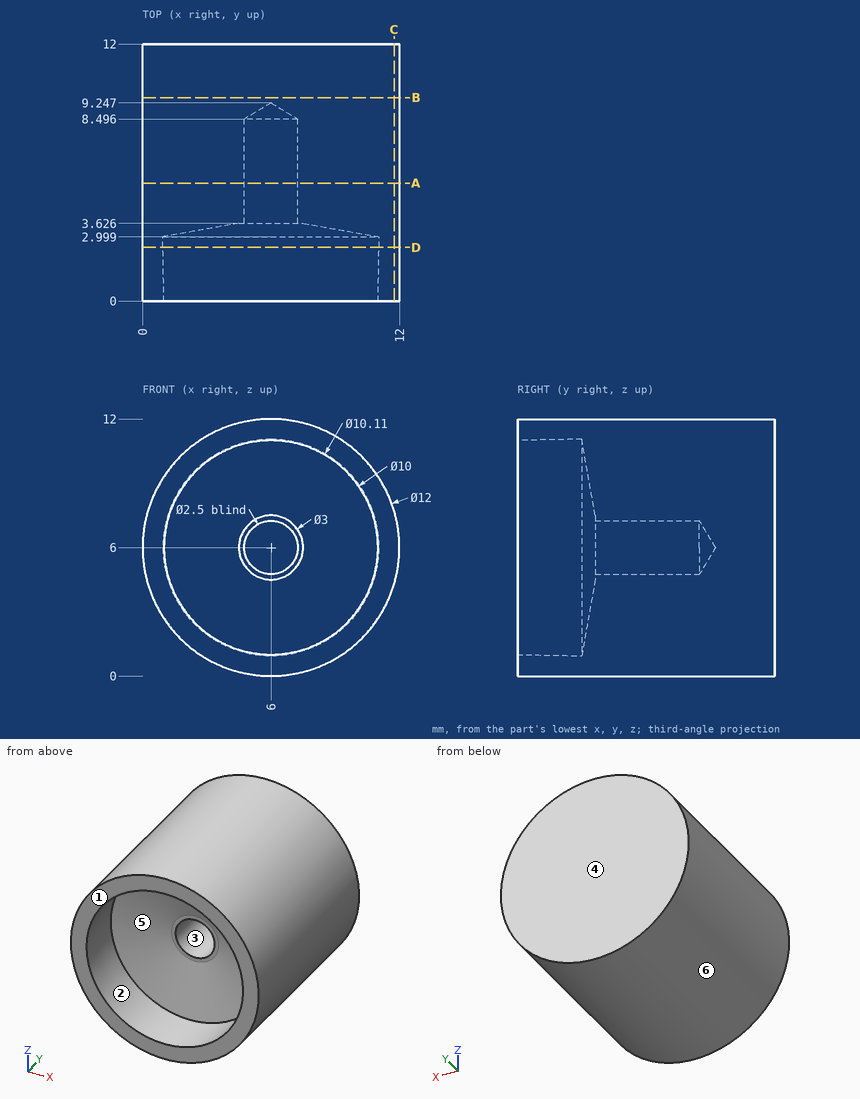
Input: dimensioned drawing with shaded views. Units: mm. Origin: part minimum x, y, z. A direction names the side the tool comes from. Coordinates: 2 decimals unless noted, no trailing zeros. Loops run counter-clockwise (first coordinate to the right, second up) from the corner with the lowest first, then second, coordinate; pieces in that order, holes last. Notation, with made-up numbers: M 74,80.5 L 85,80.5 A27 cw 85,103.5 Z; hole C 79,73 d8. An arc over 180 degrees is marked long. Use a Markdown table: item, result. Add a question column.
1) Section C-C, the plane x = 11.75. Return the cut outline in (y, z).
2) Section A-A, the plane y = 5.5. Return the cut outline in (x, z).
3) Set-up query: the marked faces 1 and 2. Return all of +Z, -Z, +X, -X, +Y, -Y with unobstructed straight access to the full face (end or side cutting, diameter ignored); none if empty.
4) Line query: L1, parallel to X at y = 5.1, z = 6; L2, parallel to X at y = 2.5, z = 10 (1 decimal). Output: solid intervals per line, ascending. Write a range as from..to.
5) Draft query along Z for the marked faces 3, 4, 5 and 6. Return one class per face: +Z half, -Z half, draft (parallel to the pull), parting line (faces both ways), or undercut.
6) Section D-D, the plane y = 2.5. Return the cut outline in (x, z) (1 decimal).
7) Section B-B, the plane y = 9.5. Return the cut outline in (x, z).
8) Pin query (flat end, axial travel): P1, Ø2.5, axis at x = 6.5, z = 6, coming from the -Y side; P2, Ø1.5, axis at x = 10, y = 6.5, coming from the +Z side (1 decimal); P3, Ø1, axis at x = 8.5, y = 1.5, coming from the -Z side. Return the tip coordinate at first contact, or that it passes through.
Answer below:
| question | item | result |
|---|---|---|
| 1 | outline | M 0,4.29 L 12,4.29 L 12,7.71 L 0,7.71 Z |
| 2 | outline | C 6,6 d12; hole C 6,6 d2.5 |
| 3 | face 1 | +Z, -Z, +X, -X, -Y |
| 3 | face 2 | none |
| 4 | L1 | 0..4.75, 7.25..12 |
| 4 | L2 | 1.5..2.9, 9.1..10.5 |
| 5 | face 3 | undercut |
| 5 | face 4 | draft |
| 5 | face 5 | undercut |
| 5 | face 6 | parting line |
| 6 | outline | C 6,6 d12; hole C 6,6 d10.1 |
| 7 | outline | C 6,6 d12 |
| 8 | P1 | y = 3.58 |
| 8 | P2 | z = 11 |
| 8 | P3 | z = 0.34 |
